from build123d import *

# Parameters (mm, degrees)
F1_DEPTH = 13
F2_R     = 1
F3_R     = 1
F4_DEPTH = 25
F5_R     = 1
F6_DEPTH = 25


with BuildPart() as f1:
    # F0 (on Front) → F1 (new body)
    with BuildSketch(Plane.XZ):
        Polygon((-20.4238126724, 0), (-18.61380395, 0), (-15.4238126724, 0), (-15.4238126724, 3), (-1.4238126724, 3), (-1.4238126724, 0), (3.5761873276, 0), (3.5761873276, 2), (0.5761873276, 2), (0.5761873276, 5), (-17.4186695367, 5), (-17.4238126724, 2), (-20.4238126724, 2), align=None)
    extrude(amount=F1_DEPTH)

    # F2
    f2_edges = [f1.edges().sort_by_distance(p)[0] for p in [
        (-8.421241, 0, 5),
        (0.576187, -6.5, 5),
        (-17.41867, -6.5, 5),
        (-8.421241, -13, 5),
        (3.576187, -6.5, 2),
        (-20.423813, -6.5, 2),
    ]]
    fillet(f2_edges, radius=F2_R)

    # F3 (on face) → F4 (cut)
    with BuildSketch(Plane(origin=(0, 0, 0), x_dir=(1, 0, 0), z_dir=(0, 0, -1))):
        with Locations((-18.4238126724, 10)):
            Circle(F3_R)
        with Locations((-18.4238126724, 3)):
            Circle(F3_R)
    extrude(amount=-F4_DEPTH, mode=Mode.SUBTRACT)

    # F5 (on face) → F6 (cut)
    with BuildSketch(Plane(origin=(0, 0, 0), x_dir=(1, 0, 0), z_dir=(0, 0, -1))):
        with Locations((1.5761873276, 10)):
            Circle(F5_R)
        with Locations((1.5761873276, 3)):
            Circle(F5_R)
    extrude(amount=-F6_DEPTH, mode=Mode.SUBTRACT)


solid = f1.part
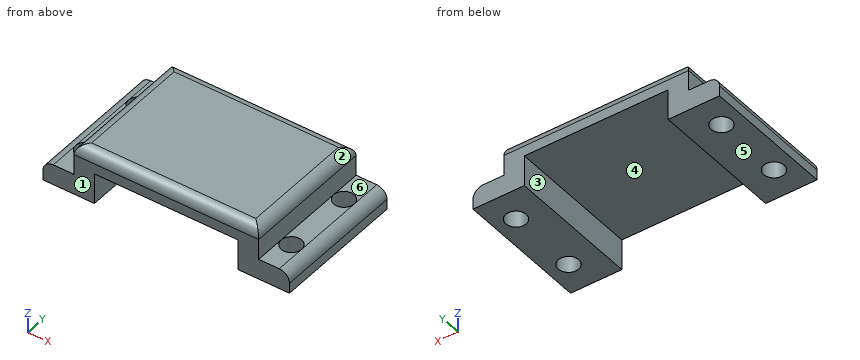
Geometry check sheet. Reference: the model listing, model coordinates, mm. Face numbers are marked on the shaded views. A direction names the side the tool comes from. Round coordinates to 2 decimals unless told otherwise and drop trailing zeros. Loops run counter-clockwise (first coordinate to the right, second up) from the corner with the lowest first, then second, coordinate; pieces in that order, holes last.
Item 1: Mould release check, pull along X, two halves, no side actions. Record for the marked faces 1, 2, 3 and 4: pulls with the +X half, pulls with the -X half, needs draft (parallel to the pull), parting line crosses it, or undercut.
Item 2: Cross-section at C-C on z = 4.65. Record the boundary of the cut face in (x, y).
Item 3: Cross-section at B-B on x = -7.5. Record the boundary of the cut face in (y, z).
Item 4: Gauge pin test, flat ends, axial feed: pin 1 (1 mm diameter, centred on x = 1.5, y = -6.5, fed in from +Z); pin 2 (6.5 mm diameter, centred on x = -8.5, y = -8.5, fed in from -Z); pin 3 (2 mm diameter, centred on x = -10.5, z = 2.5, fed in from +Y); pin 4 (0.6 mm diameter, centred on y = -7.5, z = 3.5, fed in from +X). Record the tip position at first contact, or that the pin passes through.
Item 5: Cross-section at A-A on y = -11.75. Record the boundary of the cut face in (x, z).
Item 6: Access from +Z, -Z, +X, -X, +Y, -Y to the whole of each face (thin tool, end or side, straight path). Record for the marked faces 5 and 6.
Item 7: Thickness scan on line 1 (X direction, y = -3, z = 0.6); line 2 (Y direction, x = -18.5, z = 1.65); line 3 (X direction, y = -4, z = 2.7). Record the ranges inside material, lowest first.
Answer sheet:
1. face 1: needs draft
1. face 2: pulls with the +X half
1. face 3: undercut
1. face 4: undercut
2. outline: (-17.18, -12.76) - (0.34, -12.76) - (0.34, -0.24) - (-17.18, -0.24) - close
3. outline: (-13, 3) - (0, 3) - (0, 4) arc R1 ccw to (-1, 5) - (-12, 5) arc R1 ccw to (-13, 4) - close
4. pin 1: stops at z = 2
4. pin 2: stops at z = 3
4. pin 3: stops at y = 0
4. pin 4: stops at x = 0.58
5. outline: (-20.42, 0) - (-15.42, 0) - (-15.42, 3) - (-1.42, 3) - (-1.42, 0) - (3.58, 0) - (3.58, 1) arc R1 ccw to (2.58, 2) - (0.58, 2) - (0.58, 4) arc R1 ccw to (-0.42, 5) - (-16.42, 5) arc R1 ccw to (-17.42, 4) - (-17.42, 2) - (-19.42, 2) arc R1 ccw to (-20.42, 1) - close
6. face 5: -Z, +X, -X, +Y, -Y
6. face 6: +Z, +X, +Y, -Y
7. line 1: x = -20.42 to -19.42, -17.42 to -15.42, -1.42 to 0.58, 2.58 to 3.58
7. line 2: y = -13 to -11, -9 to -4, -2 to 0
7. line 3: x = -17.42 to -15.42, -1.42 to 0.58
